Geometry: final body of the model. Coordinates: model frame, mm. A direction names the side the tool comes from. Coordinates: 2 decimals unless noted, no trailing zeros. One line per item, written item: value. Start each with the question number.
Item 1: Mould query, pull axis Y, two halves, no side actions, for faces 4 (the cylindrical face through (1.11, 9, 19.57)), 5 (the flat face through (1, 7.5, 10)), 6 (the flat face through (80, 11, 8)). Classes: +Y half, -Y half, draft (parallel to the pull), parting line (faces both ways), or undercut.
Item 2: Ray query, probe 1 along Y at (x, z) = (19, -2); probe 2 along Y at (x, z) = (-53, 14.25); probe 3 along Y at (x, z) = (-33.5, 16.5). Return the intervals inside material, ascending. Write a range as from..to.
Item 3: Set-up query: faces 1 (the cylindrical face through (1.11, -8.94, 9.51)), 2 (the flat face through (38, 1.5, -5)), 3 (the flat face through (1, 15, 21)). Return all of +Z, -Z, +X, -X, +Y, -Y with unobstructed straight access to the full face (end or side cutting, diameter ignored); none if empty.
Item 4: Contact query for flat-ended pins moving along their axis: pin 1 Ø2 at (y, z) = (-2.5, -3.5) entering from -X; pin 2 Ø2 at (y, z) = (-9.5, -2.5) entering from +X; pin 3 Ø0.8 at (x, y) = (38, 3) entering from +Z. Output: stop coordinate, or through.
from build123d import *

# Parameters (mm, degrees)
F1_DEPTH  = 80
F2_W      = 156
F2_H      = 31
F3_DEPTH  = 2
F4_W      = 5
F4_H      = 5
F5_DEPTH  = 2.2
F6_W      = 5
F6_H      = 7
F7_DEPTH  = 2
F8_W      = 5
F8_H      = 3
F9_DEPTH  = 4.2
F10_R     = 1.99999
F11_W     = 20
F11_H     = 7
F12_DEPTH = 2
F13_R     = 3
F14_R     = 0.99999


# Not quite as in the source:
# - a fillet or chamfer is up to 0.001 mm smaller than in the source, because OpenCascade refuses the exact size


with BuildPart() as f1:
    # F0 (on Right) → F1 (new body, symmetric)
    with BuildSketch(Plane.YZ):
        with BuildLine():
            Line((7.5, 1), (17.5, 1))
            Line((17.5, 1), (17.5, 21))
            Line((17.5, 21), (12.5, 21))
            ThreePointArc((12.5, 21), (8.9644660941, 19.5355339059), (7.5, 16))
            Line((7.5, 16), (7.5, 1))
        make_face()
        Polygon((17.5, -1), (17.5, 1), (7.5, 1), (-2.5, 1), (-7.5, 1), (-12.5, 1), (-17.5, 1), (-17.5, -1), align=None)
        with BuildLine():
            Line((-17.5, 16), (-17.5, 1))
            Line((-17.5, 1), (-12.5, 1))
            Line((-12.5, 1), (-12.5, 11))
            ThreePointArc((-12.5, 11), (-13.9644660941, 14.5355339059), (-17.5, 16))
        make_face()
        with BuildLine():
            Line((-12.5, 1), (-7.5, 1))
            Line((-7.5, 1), (-7.5, 6))
            ThreePointArc((-7.5, 6), (-8.9644660941, 9.5355339059), (-12.5, 11))
            Line((-12.5, 11), (-12.5, 1))
        make_face()
        with BuildLine():
            Line((-7.5, 1), (-2.5, 1))
            ThreePointArc((-2.5, 1), (-3.9644660941, 4.5355339059), (-7.5, 6))
            Line((-7.5, 6), (-7.5, 1))
        make_face()
    extrude(amount=F1_DEPTH, both=True)

    # F2 (on face) → F3 (join)
    with BuildSketch(Plane(origin=(0, 0, -1), x_dir=(1, 0, 0), z_dir=(0, 0, -1))):
        Rectangle(F2_W, F2_H)
    extrude(amount=F3_DEPTH)

    # F4 (on face) → F5 (join)
    with BuildSketch(Plane(origin=(0, 0, -3), x_dir=(1, 0, 0), z_dir=(0, 0, -1))):
        with Locations((38, 0)):
            Rectangle(F4_W, F4_H)
    extrude(amount=F5_DEPTH)

    # F6 (on face) → F7 (join)
    with BuildSketch(Plane(origin=(0, 0, -5.2), x_dir=(1, 0, 0), z_dir=(0, 0, -1))):
        with Locations((38, 0)):
            Rectangle(F6_W, F6_H)
    extrude(amount=F7_DEPTH)

    # F8 (on face) → F9 (cut)
    with BuildSketch(Plane(origin=(0, 0, -7.2), x_dir=(1, 0, 0), z_dir=(0, 0, -1))):
        with Locations((38, 0)):
            Rectangle(F8_W, F8_H)
    extrude(amount=-F9_DEPTH, mode=Mode.SUBTRACT)

    # F10 (radius 2 in the source; OpenCascade refuses exactly that, so slightly less here)
    f10_edges = [f1.edges().sort_by_distance(p)[0] for p in [
        (40.5, 2.5, -7.2),
        (38, 3.5, -7.2),
        (40.5, -2.5, -7.2),
        (38, -3.5, -7.2),
        (35.5, -2.5, -7.2),
        (35.5, 2.5, -7.2),
    ]]
    fillet(f10_edges, radius=F10_R)

    # F11 (on face) → F12 (cut)
    with BuildSketch(Plane(origin=(0, 0, -3), x_dir=(1, 0, 0), z_dir=(0, 0, -1))):
        with Locations((68, 0)):
            Rectangle(F11_W, F11_H)
    extrude(amount=-F12_DEPTH, mode=Mode.SUBTRACT)

    # F13
    f13_edges = [f1.edges().sort_by_distance(p)[0] for p in [
        (0, -12.5, 11),
        (0, -7.5, 6),
        (0, -2.5, 1),
        (0, 7.5, 1),
    ]]
    fillet(f13_edges, radius=F13_R)

    # F14 (radius 1 in the source; OpenCascade refuses exactly that, so slightly less here)
    f14_edges = [f1.edges().sort_by_distance(p)[0] for p in [
        (80, 7.5, 10),
        (80, 6.62132, 1.87868),
        (80, 8.964466, 19.535534),
        (80, 2.208099, 1),
        (80, 15, 21),
        (80, -1.760852, 1.512531),
        (80, 17.5, 10),
        (80, -4.066216, 4.634436),
        (80, 0, -1),
        (80, -7.046875, 6.453125),
        (80, -17.5, 7.5),
        (80, -8.964466, 9.535534),
        (80, -14.588398, 15.064797),
        (80, -12.046875, 11.453125),
        (-80, 7.5, 10),
        (-80, 6.62132, 1.87868),
        (-80, 8.964466, 19.535534),
        (-80, 2.208099, 1),
        (-80, 15, 21),
        (-80, -1.760852, 1.512531),
        (-80, 17.5, 10),
        (-80, -4.066216, 4.634436),
        (-80, 0, -1),
        (-80, -7.046875, 6.453125),
        (-80, -17.5, 7.5),
        (-80, -8.964466, 9.535534),
        (-80, -14.588398, 15.064797),
        (-80, -12.046875, 11.453125),
    ]]
    fillet(f14_edges, radius=F14_R)


solid = f1.part
Reply:
1. face 4: -Y half
1. face 5: undercut
1. face 6: draft
2. probe 1: y = -15.5..15.5
2. probe 2: y = -17.5..-13.7, 7.5..17.5
2. probe 3: y = 7.53..17.5
3. face 1: +Z, +X, -X
3. face 2: -Z, +X, -X
3. face 3: +Z, +X, -X, +Y, -Y
4. pin 1: stops at x = -78
4. pin 2: stops at x = 78
4. pin 3: stops at z = 1
